```python
from build123d import *

# Parameters (mm, degrees)
SKETCH1_W           = 140
SKETCH1_H           = 72
BOSS_EXTRUDE1_DEPTH = 17
SKETCH2_R           = 34.1
CUT_EXTRUDE1_DEPTH  = 12
SKETCH3_W           = 40
SKETCH3_H           = 24
CUT_EXTRUDE2_DEPTH  = 10
SKETCH4_R           = 2.2
CUT_EXTRUDE3_DEPTH  = 81.529497701
SKETCH5_R           = 2.25
SKETCH5_R_2         = 4.5
CUT_EXTRUDE4_DEPTH  = 80.62411695
CUT_EXTRUDE5_DEPTH  = 10


with BuildPart() as part:
    # Sketch1 → Boss-Extrude1 (new body)
    with BuildSketch(Plane(origin=(0, 0, 0), x_dir=(1, 0, 0), z_dir=(0, 1, 0))):
        Rectangle(SKETCH1_W, SKETCH1_H)
    extrude(amount=BOSS_EXTRUDE1_DEPTH)

    # Sketch2 → Cut-Extrude1 (cut)
    with BuildSketch(Plane(origin=(0, 17, 0), x_dir=(1, 0, 0), z_dir=(0, 1, 0))):
        with Locations(Location((0, 0, 0), (0, 0, 270))):
            Circle(SKETCH2_R)
    extrude(amount=-CUT_EXTRUDE1_DEPTH, mode=Mode.SUBTRACT)

    # Sketch3 → Cut-Extrude2 (cut)
    with BuildSketch(Plane.XY.offset(36)):
        with Locations((0, 17)):
            Rectangle(SKETCH3_W, SKETCH3_H)
    extrude(amount=-CUT_EXTRUDE2_DEPTH, mode=Mode.SUBTRACT)

    # Sketch4 → Cut-Extrude3 (cut, through all)
    with BuildSketch(Plane(origin=(0, 17, 0), x_dir=(1, 0, 0), z_dir=(0, 1, 0))):
        with Locations(Location((-62.5, 25, 0), (0, 0, 270))):
            Circle(SKETCH4_R)
        with Locations(Location((-62.5, 0, 0), (0, 0, 270))):
            Circle(SKETCH4_R)
        with Locations(Location((-62.5, -25, 0), (0, 0, 270))):
            Circle(SKETCH4_R)
        with Locations(Location((62.5, -25, 0), (0, 0, 90))):
            Circle(SKETCH4_R)
        with Locations(Location((62.5, 0, 0), (0, 0, 90))):
            Circle(SKETCH4_R)
        with Locations(Location((62.5, 25, 0), (0, 0, 90))):
            Circle(SKETCH4_R)
    extrude(amount=-CUT_EXTRUDE3_DEPTH, mode=Mode.SUBTRACT)

    # Sketch5 → Cut-Extrude4 (cut, through all)
    with BuildSketch(Plane(origin=(0, 5, 0), x_dir=(1, 0, 0), z_dir=(0, 1, 0))):
        with Locations(Location((0, 29, 0), (0, 0, 270))):
            Circle(SKETCH5_R)
        with Locations(Location((25.042343364, -14.374611046, 0), (0, 0, 270))):
            Circle(SKETCH5_R)
        with Locations(Location((-25.042343364, -14.374611046, 0), (0, 0, 270))):
            Circle(SKETCH5_R)
        with Locations(Location((0, 19.333592636, 0), (0, 0, 270))):
            Circle(SKETCH5_R_2)
    extrude(amount=-CUT_EXTRUDE4_DEPTH, mode=Mode.SUBTRACT)

    # Sketch6 → Cut-Extrude5 (cut)
    with BuildSketch(Plane(origin=(0, 17, 0), x_dir=(1, 0, 0), z_dir=(0, 1, 0))):
        with BuildLine():
            Line((-55, 31), (-25.27844932, 31))
            ThreePointArc((-25.27844932, 31), (-37.491645865, 13.941896942), (-39.391334679, -6.951456838))
            Line((-39.391334679, -6.951456838), (-55, 19.35498509))
            Line((-55, 19.35498509), (-55, 31))
        make_face()
        with BuildLine():
            Line((-55, -31), (-25.27844932, -31))
            ThreePointArc((-25.27844932, -31), (-30.757821307, -25.5725718), (-35.093761786, -19.194475343))
            Line((-35.093761786, -19.194475343), (-55, 14.35498509))
            Line((-55, 14.35498509), (-55, -31))
        make_face()
        with BuildLine():
            Line((55, -31), (25.27844932, -31))
            ThreePointArc((25.27844932, -31), (30.757821307, -25.5725718), (35.093761786, -19.194475343))
            Line((35.093761786, -19.194475343), (55, 14.35498509))
            Line((55, 14.35498509), (55, -31))
        make_face()
        with BuildLine():
            Line((55, 31), (55, 19.35498509))
            Line((55, 19.35498509), (39.391334679, -6.951456838))
            ThreePointArc((39.391334679, -6.951456838), (37.491645865, 13.941896942), (25.27844932, 31))
            Line((25.27844932, 31), (55, 31))
        make_face()
    extrude(amount=-CUT_EXTRUDE5_DEPTH, mode=Mode.SUBTRACT)


solid = part.part
```
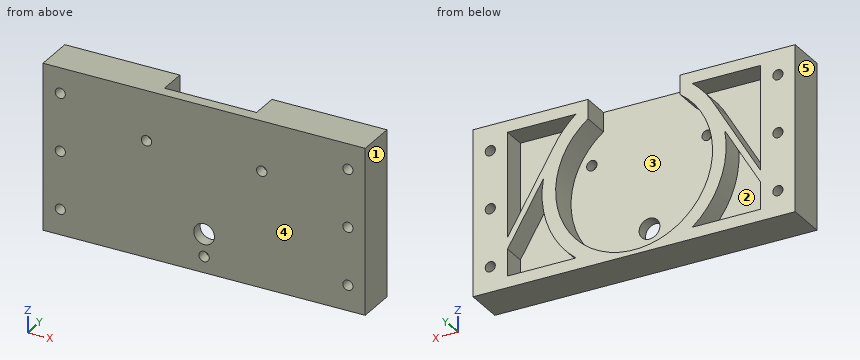
Geometry check sheet. Reference: the model listing, model coordinates, mm. Face numbers are marked on the shaded views. A direction names the side the tool comes from. Round coordinates to 2 decimals unless told otherwise and drop trailing zeros. Loops run counter-clockwise (first coordinate to the right, second up) from the corner with the lowest first, then second, coordinate; pieces in that order, holes last. Notation, with made-up numbers: (-8.5, -39.75) - (43.5, -39.75) arc R27 cw to (43.5, -20.75) - close; hole circle Ø10 at (69.25, 72). An arc over 180 degrees is marked (long way). Write each question's results on one line, items separated by ' | '. Start each with the question number.
Q1. Thickness scan on line 1 (X direction, y = 4.25, z = 25); line 2 (Z direction, x = 62.5, y = 13.25); line 3 (X direction, y = 14, z = 21). Record the ranges inside material, lowest first. Write a range as [from, to].
Q2. Gauge pin test, flat ends, axial feed: P1, Ø5, axis at x = 39.5, z = -25.5, coming from the +Y side; P2, Ø12, axis at x = -23.5, z = -25, coming from the -Y side; P3, Ø5.5, axis at x = 0, z = -19.33, coming from the +Y side; P4, Ø2, axis at x = -19.5, z = 8, coming from the +Y side. Record the tip position at first contact, or that the pin passes through.
Q3. Cross-section at A-A on y = 8.5. State how many separate pieces and enclosed holes the cut face has, and give its area (3 significant figures).
Q4. Cross-section at C-C on z = -29. Enter the section's corners in (x, y), and give its area (3 significant figures).
Q5. Release check for a two-part mould opening along X. For the marked faces 3, 4 and 5 record: +X half, -X half, draft (parallel to the pull), parting line (faces both ways), or undercut.
Q6. Access from +Z, -Z, +X, -X, +Y, -Y to the whole of each face (thin tool, end or side, straight path). Record for the marked faces 1 and 2.
Q7. Cross-section at D-D on x = -32. Enter the section's corners in (y, z), and give its area (3 significant figures).
Answers below:
1) line 1: x = [-70, -64.7], [-60.3, 60.3], [64.7, 70] | line 2: z = [-36, -27.2], [-22.8, -2.2], [2.2, 22.8], [27.2, 36] | line 3: x = [-70, -55], [-34.04, -26.87], [26.87, 34.04], [55, 70]
2) P1: stops at y = 7 | P2: stops at y = 0 | P3: passes through | P4: stops at y = 5
3) separate pieces: 1 | enclosed holes: 10 | area: 3,930 mm²
4) outline: (-70, 0) - (-2.25, 0) - (-2.25, 5) - (-17.94, 5) - (-17.94, 17) - (-27.55, 17) - (-27.55, 7) - (-55, 7) - (-55, 17) - (-70, 17) - close; (2.25, 0) - (70, 0) - (70, 17) - (55, 17) - (55, 7) - (27.55, 7) - (27.55, 17) - (17.94, 17) - (17.94, 5) - (2.25, 5) - close | area: 1,380 mm²
5) face 3: undercut | face 4: draft | face 5: -X half
6) face 1: +Z, -Z, +X, +Y, -Y | face 2: +Y
7) outline: (0, -36) - (17, -36) - (17, -31) - (7, -31) - (7, -24) - (17, -24) - (17, -11.78) - (5, -11.78) - (5, 11.78) - (17, 11.78) - (17, 24) - (7, 24) - (7, 31) - (17, 31) - (17, 36) - (0, 36) - close | area: 801 mm²
